Could you check a few things on this model? Use its own coordinates, in mm. A direction names the side the tool comes from. Round coordinates to 2 decimals unless told otherwise and drop trailing zeros. One line per item, written item: value. Start each with the question number.
(1) If I drill on L1, parallel to X at y = 58.5, z = -67; L2, parallel to X at y = 60, z = 18.5; L3, parallel to Z at x = 40.5, y = 57.75, over which ranges is the centre line in solid material (lowest first)?
(2) Thinking about a two-plate mould opening in X: for faces 3 (the face through (60.789, 60.07, -78.085)), 4 (the face through (6, 60, -79.889)), 5 (the face through (41.354, 60.711, -68.237)), 6 (the face through (-42.428, 62.776, 20.055)), which applies, released by +X, released by -X, zero draft, split by the parting line, or undercut?
(3) Which directions (+Z, -Z, +X, -X, +Y, -Y) give clear straight access to the entire face, cutting with the end or side of a thin tool? Please do faces 1 (the face through (52.865, 62.776, 20.055)), 2 (the face through (6, 55, -27)).
(4) I'm going to push flat-ended pins straight in: pin 1 Ø4.5 at (x, y) = (-42.79, 60) entering from +Z; pin 2 Ø4.5 at (x, z) = (41.54, -66.8) entering from -Y. Where does each tip first touch, or does it pass through?
```python
from build123d import *

# Parameters (mm, degrees)
SKETCH2_W                                         = 115.292618629
SKETCH2_H                                         = 134.000000002
BOSS_EXTRUDE2_DEPTH                               = 8
FILLET2_R                                         = 6
SKETCH19_W                                        = 8
SKETCH19_H                                        = 99
BOSS_EXTRUDE3_DEPTH                               = 115.292618629
SKETCH21_W                                        = 135.292618629
SKETCH21_H                                        = 129
SKETCH21_W_2                                      = 115.292618629
SKETCH21_H_2                                      = 99
BOSS_EXTRUDE4_DEPTH                               = 8
FILLET3_R                                         = 5
CUT_EXTRUDE1_DEPTH                                = 4
SKETCH24_W                                        = 115.292618629
SKETCH24_H                                        = 10
BOSS_EXTRUDE5_DEPTH                               = 104
FILLET4_R                                         = 6
CSK_FOR_M2_5_FLAT_HEAD_MACHINE_SCREW2_D           = 2.9
CSK_FOR_M2_5_FLAT_HEAD_MACHINE_SCREW2_DEPTH       = 10
CSK_FOR_M2_5_FLAT_HEAD_MACHINE_SCREW2_CSINK_D     = 5.5
CSK_FOR_M2_5_FLAT_HEAD_MACHINE_SCREW2_CSINK_ANGLE = 90
SKETCH49_R                                        = 4.43
CUT_EXTRUDE3_DEPTH                                = 8
M2_5_CLEARANCE_HOLE1_D                            = 2.9
CUT_EXTRUDE4_START                                = -8
CUT_EXTRUDE4_DEPTH                                = 8
CHAMFER1_SIZE                                     = 0.9
SKETCH62_W                                        = 134.000000002
SKETCH62_H                                        = 8
CUT_EXTRUDE5_DEPTH                                = 115.292618629
SKETCH63_W                                        = 135.292618629
SKETCH63_H                                        = 8
CUT_EXTRUDE6_DEPTH                                = 129
F_5_6_5_6_DIAMETER_HOLE1_D                        = 5.6
F_5_6_5_6_DIAMETER_HOLE1_DEPTH                    = 8
F_5_6_5_6_DIAMETER_HOLE1_TIP                      = 1.682409733


with BuildPart() as part:
    # Sketch2 → Boss-Extrude2 (new body)
    with BuildSketch(Plane(origin=(0, 0, 0), x_dir=(1, 0, 0), z_dir=(0, 1, 0))):
        with Locations((4.853690686, 42.889279439)):
            Rectangle(SKETCH2_W, SKETCH2_H)
    extrude(amount=BOSS_EXTRUDE2_DEPTH)

    # Fillet2
    fillet2_edges = [part.edges().sort_by_distance(p)[0] for p in [
        (-52.792618629, 4, -109.88927944),
        (62.5, 4, -109.88927944),
    ]]
    fillet(fillet2_edges, radius=FILLET2_R)

    # Sketch19 → Boss-Extrude3 (add)
    with BuildSketch(Plane.ZY.offset(52.792618629)):
        with Locations((28.110720562, 13.5)):
            Rectangle(SKETCH19_W, SKETCH19_H)
    extrude(amount=-BOSS_EXTRUDE3_DEPTH)

    # Sketch21 → Boss-Extrude4 (add)
    with BuildSketch(Plane.XY.offset(32.110720562)):
        with Locations((4.853690685, 8.5)):
            Rectangle(SKETCH21_W, SKETCH21_H)
        with Locations((4.853690686, 13.5)):
            Rectangle(SKETCH21_W_2, SKETCH21_H_2, mode=Mode.SUBTRACT)
    extrude(amount=-BOSS_EXTRUDE4_DEPTH)

    # Fillet3
    fillet3_edges = [part.edges().sort_by_distance(p)[0] for p in [
        (72.5, 73, 28.110720562),
        (72.5, -56, 28.110720562),
        (-62.792618629, -56, 28.110720562),
        (-62.792618629, 73, 28.110720562),
    ]]
    fillet(fillet3_edges, radius=FILLET3_R)

    # Sketch22 → Cut-Extrude1 (cut)
    with BuildSketch(Plane(origin=(0, 0, 24.110720562), x_dir=(-1, 0, 0), z_dir=(0, 0, -1))):
        with BuildLine():
            Line((62.792618629, -51), (62.792618629, 68))
            ThreePointArc((62.792618629, 68), (61.328152535, 71.535533906), (57.792618629, 73))
            Line((57.792618629, 73), (-67.5, 73))
            ThreePointArc((-67.5, 73), (-71.035533906, 71.535533906), (-72.5, 68))
            Line((-72.5, 68), (-72.5, -51))
            ThreePointArc((-72.5, -51), (-71.035533906, -54.535533906), (-67.5, -56))
            Line((-67.5, -56), (57.792618629, -56))
            ThreePointArc((57.792618629, -56), (61.328152535, -54.535533906), (62.792618629, -51))
        make_face()
        with BuildLine():
            Line((57.792618629, 69.75), (-67.5, 69.75))
            ThreePointArc((-67.5, 69.75), (-68.737436867, 69.237436867), (-69.25, 68))
            Line((-69.25, 68), (-69.25, -51))
            ThreePointArc((-69.25, -51), (-68.737436867, -52.237436867), (-67.5, -52.75))
            Line((-67.5, -52.75), (57.792618629, -52.75))
            ThreePointArc((57.792618629, -52.75), (59.030055496, -52.237436867), (59.542618629, -51))
            Line((59.542618629, -51), (59.542618629, 68))
            ThreePointArc((59.542618629, 68), (59.030055496, 69.237436867), (57.792618629, 69.75))
        make_face(mode=Mode.SUBTRACT)
    extrude(amount=-CUT_EXTRUDE1_DEPTH, mode=Mode.SUBTRACT)

    # Sketch24 → Boss-Extrude5 (add)
    with BuildSketch(Plane(origin=(0, 0, 24.110720562), x_dir=(-1, 0, 0), z_dir=(0, 0, -1))):
        with Locations((-4.853690686, 60)):
            Rectangle(SKETCH24_W, SKETCH24_H)
    extrude(amount=BOSS_EXTRUDE5_DEPTH)

    # Fillet4
    fillet4_edges = [part.edges().sort_by_distance(p)[0] for p in [
        (62.5, 60, -79.889279438),
        (-52.792618629, 60, -79.889279438),
    ]]
    fillet(fillet4_edges, radius=FILLET4_R)

    # CSK for M2.5 Flat Head Machine Screw2
    with Locations(Plane(origin=(0, 55, 0), x_dir=(-1, 0, 0), z_dir=(0, -1, 0))):
        with Locations((16.187618629, 66.799279438), (-41.542381371, 66.799279438), (16.187618629, 17.789279438), (-41.542381371, 17.789279438)):
            CounterSinkHole(CSK_FOR_M2_5_FLAT_HEAD_MACHINE_SCREW2_D / 2, CSK_FOR_M2_5_FLAT_HEAD_MACHINE_SCREW2_CSINK_D / 2, depth=CSK_FOR_M2_5_FLAT_HEAD_MACHINE_SCREW2_DEPTH, counter_sink_angle=CSK_FOR_M2_5_FLAT_HEAD_MACHINE_SCREW2_CSINK_ANGLE)

    # Sketch49 → Cut-Extrude3 (cut)
    with BuildSketch(Plane.XY.offset(32.110720562)):
        with Locations((4.853690685, 40.159632183)):
            Circle(SKETCH49_R)
    extrude(amount=-CUT_EXTRUDE3_DEPTH, mode=Mode.SUBTRACT)

    # M2.5 Clearance Hole1 (through all)
    with Locations(Plane(origin=(0, 8, 0), x_dir=(1, 0, 0), z_dir=(0, 1, 0))):
        with Locations((-28.27, 101.64), (-7.29, 101.64), (-7.29, 88.14), (-28.27, 88.14)):
            Hole(M2_5_CLEARANCE_HOLE1_D / 2)

    # Sketch60 → Cut-Extrude4 (cut)
    with BuildSketch(Plane(origin=(0, 8, 0), x_dir=(1, 0, 0), z_dir=(0, 1, 0)).offset(CUT_EXTRUDE4_START)):
        with BuildLine():
            Line((-30.27, 103.09), (-26.27, 103.09))
            ThreePointArc((-26.27, 103.09), (-24.82, 101.64), (-26.27, 100.19))
            Line((-26.27, 100.19), (-30.27, 100.19))
            ThreePointArc((-30.27, 100.19), (-31.72, 101.64), (-30.27, 103.09))
        make_face()
        with BuildLine():
            Line((-9.29, 103.09), (-5.29, 103.09))
            ThreePointArc((-5.29, 103.09), (-3.84, 101.64), (-5.29, 100.19))
            Line((-5.29, 100.19), (-9.29, 100.19))
            ThreePointArc((-9.29, 100.19), (-10.74, 101.64), (-9.29, 103.09))
        make_face()
        with BuildLine():
            Line((-30.27, 89.59), (-26.27, 89.59))
            ThreePointArc((-26.27, 89.59), (-24.82, 88.14), (-26.27, 86.69))
            Line((-26.27, 86.69), (-30.27, 86.69))
            ThreePointArc((-30.27, 86.69), (-31.72, 88.14), (-30.27, 89.59))
        make_face()
        with BuildLine():
            Line((-9.29, 89.59), (-5.29, 89.59))
            ThreePointArc((-5.29, 89.59), (-3.84, 88.14), (-5.29, 86.69))
            Line((-5.29, 86.69), (-9.29, 86.69))
            ThreePointArc((-9.29, 86.69), (-10.74, 88.14), (-9.29, 89.59))
        make_face()
    extrude(amount=CUT_EXTRUDE4_DEPTH, mode=Mode.SUBTRACT)

    # Chamfer1
    chamfer1_edges = [part.edges().sort_by_distance(p)[0] for p in [
        (-7.29, 8, -100.19),
        (-3.84, 8, -101.64),
        (-7.29, 8, -103.09),
        (-28.27, 8, -86.69),
        (-24.82, 8, -88.14),
        (-28.27, 8, -89.59),
        (-7.29, 8, -86.69),
        (-3.84, 8, -88.14),
        (-7.29, 8, -89.59),
        (-28.27, 8, -103.09),
        (-31.72, 8, -101.64),
        (-28.27, 8, -100.19),
        (-24.82, 8, -101.64),
        (-10.74, 8, -88.14),
        (-31.72, 8, -88.14),
        (-10.74, 8, -101.64),
    ]]
    chamfer(chamfer1_edges, length=CHAMFER1_SIZE)

    # Sketch62 → Cut-Extrude5 (cut)
    with BuildSketch(Plane.ZY.offset(52.792618629)):
        with Locations((-42.889279439, 4)):
            Rectangle(SKETCH62_W, SKETCH62_H)
    extrude(amount=-CUT_EXTRUDE5_DEPTH, mode=Mode.SUBTRACT)

    # Sketch63 → Cut-Extrude6 (cut)
    with BuildSketch(Plane(origin=(0, 73, 0), x_dir=(1, 0, 0), z_dir=(0, 1, 0))):
        with Locations((4.853690685, -28.110720562)):
            Rectangle(SKETCH63_W, SKETCH63_H)
    extrude(amount=-CUT_EXTRUDE6_DEPTH, mode=Mode.SUBTRACT)

    # Ø5.6 (5.6) Diameter Hole1
    with Locations(Plane.XY.offset(24.110720562)):
        with Locations((-42.792618629, 60), (52.5, 60)):
            Hole(F_5_6_5_6_DIAMETER_HOLE1_D / 2, depth=F_5_6_5_6_DIAMETER_HOLE1_DEPTH)
            with Locations((0, 0, -(F_5_6_5_6_DIAMETER_HOLE1_DEPTH + F_5_6_5_6_DIAMETER_HOLE1_TIP / 2))):  # 118° drill point
                Cone(0, F_5_6_5_6_DIAMETER_HOLE1_D / 2, F_5_6_5_6_DIAMETER_HOLE1_TIP, mode=Mode.SUBTRACT)


solid = part.part
```
Found:
1. L1: x = -52.79 to -17.62, -14.75 to 40.11, 42.98 to 62.5
1. L2: x = -52.79 to -45.59, -39.99 to 49.7, 55.3 to 62.5
1. L3: z = -79.89 to -67.81, -65.79 to -18.8, -16.78 to 24.11
2. face 3: released by +X
2. face 4: zero draft
2. face 5: undercut
2. face 6: undercut
3. face 1: +Z
3. face 2: +Z, -Z, +X, -X, -Y
4. pin 1: stops at z = 15.78
4. pin 2: stops at y = 55.5
